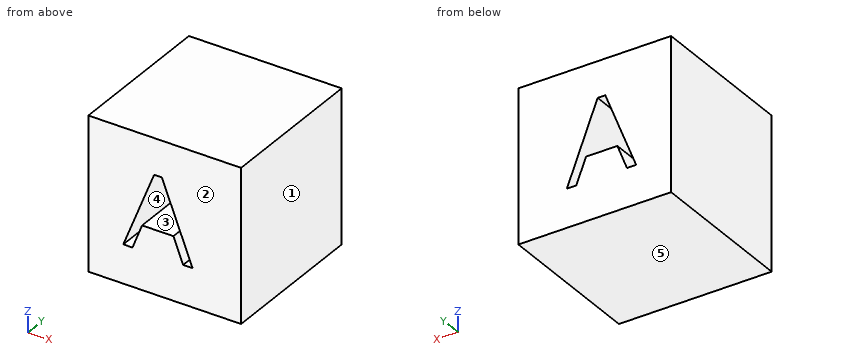
```python
from build123d import *

# Parameters (mm, degrees)
F0_W     = 50.8
F0_H     = 50.8
F1_DEPTH = 25.4


with BuildPart() as f1:
    # F0 (on Front) → F1 (new body, symmetric)
    with BuildSketch(Plane.XZ):
        with Locations((2.5065707316, 0)):
            Rectangle(F0_W, F0_H)
        Polygon((11.7624275368, -12.6344077289), (8.6336481415, -12.6344077289), (5.3967836399, -4.3687414355), (-5.0192074016, -4.3687414355), (-8.2162510746, -12.6344077289), (-11.2767661922, -12.6344077289), (-1.002992396, 13.4653011177), (1.5398519489, 13.4653011177), align=None, mode=Mode.SUBTRACT)
    extrude(amount=F1_DEPTH, both=True)


solid = f1.part
```
Geometry: final body of the model. Coordinates: model frame, mm. Face numbers are marked on the shaded views. A direction names the side the tool comes from. Round coordinates to 2 decimals unless told otherwise and drop trailing zeros. Loops run counter-clockwise (first coordinate to the right, second up) from the corner with the lowest first, then second, coordinate; pieces in that order, holes last. Notation, with made-up numbers: (57, 60) -> (96, 60) arc R21 ccw to (96, 75) -> close; hole circle Ø6 at (77.25, -12). An arc over 180 degrees is marked (long way). Use one line per item in the form item = value. Start each with the question number.
1) Section A-A on x = -7.5. Output: boundary loops of the cut face in (y, z), then the cut area to 3 significant figures.
2) Section B-B on y = -8.5. Output: boundary loops of the cut face in (x, z).
3) Access query for the marked faces 4 and 5. Directions: +Z, -Z, +X, -X, +Y, -Y. A direction counts if a zero-diameter tool reaches every point of the face in a straight line with its end or side. Return the directions, or none.
4) Section C-C on z = 1.5. Output: boundary loops of the cut face in (x, y).
5) Line query: L1, parallel to X at y = 15.5, z = -6; L2, parallel to X at y = 16, z = -10.5; L3, parallel to X at y = 21, z = 3. Output: solid intervals per line, ascending.
6) Draft query along X for the marked faces 1, 2 and 3. Return one class per face: released by +X, released by -X, zero draft, split by the parting line, or undercut.
Response:
q1.outline = (-25.4, -25.4) -> (25.4, -25.4) -> (25.4, -10.78) -> (-25.4, -10.78) -> close; (-25.4, -3.04) -> (25.4, -3.04) -> (25.4, 25.4) -> (-25.4, 25.4) -> close
q1.area = 2,190 mm^2
q2.outline = (-22.89, -25.4) -> (27.91, -25.4) -> (27.91, 25.4) -> (-22.89, 25.4) -> close; hole (-11.28, -12.63) -> (-8.22, -12.63) -> (-5.02, -4.37) -> (5.4, -4.37) -> (8.63, -12.63) -> (11.76, -12.63) -> (1.54, 13.47) -> (-1, 13.47) -> close
q3.face_4 = +Y, -Y
q3.face_5 = -Z, +X, -X, +Y, -Y
q4.outline = (-22.89, -25.4) -> (-5.71, -25.4) -> (-5.71, 25.4) -> (-22.89, 25.4) -> close; (6.23, -25.4) -> (27.91, -25.4) -> (27.91, 25.4) -> (6.23, 25.4) -> close
q5.L1 = -22.89 to -8.67, -5.65 to 6.04, 9.16 to 27.91
q5.L2 = -22.89 to -10.44, -7.39 to 7.8, 10.93 to 27.91
q5.L3 = -22.89 to -5.12, 5.64 to 27.91
q6.face_1 = released by +X
q6.face_2 = zero draft
q6.face_3 = undercut
